Could you check a few things on this model? Use its own coordinates, in mm. Face numbers are marked on the shaded views. A direction names the side the tool comes from. Give positions to 0.01 mm unless a question says otherwise; leave off trailing zeros. Write each loop counter-clockwise with the first axis right and the second up, starting at its lowest first coordinate (ties: lowest second). Pieces come first, ordered by that corner, then holes. Notation, with made-up numbers: (40, -2) - (54, -2) arc R32 cw to (54, 34) - close; hole circle Ø5 at (-6, 86). An arc over 180 degrees is marked (long way). Answer in a Markdown table with one row per item.
from build123d import *

# Parameters (mm, degrees)
F2_R     = 4.7625
F2_R_2   = 1.5875
F5_DEPTH = 3.175
F6_DEPTH = 3.175
F4_W     = 7.239
F4_H     = 4.654424265
F7_DEPTH = 1.5875
F8_SIZE  = 0.79375


with BuildPart() as f5:
    # F2 (on offset) → F5 (new body, symmetric)
    with BuildSketch(Plane.XZ.offset(25.4)):
        Circle(F2_R)
        Circle(F2_R_2, mode=Mode.SUBTRACT)
    extrude(amount=F5_DEPTH, both=True)

    # F3 (on offset) → F6 (join, symmetric)
    with BuildSketch(Plane.XZ.offset(25.4)):
        with BuildLine():
            Line((3.175, 0), (3.175, 12.7))
            Line((3.175, 12.7), (-3.175, 12.7))
            Line((-3.175, 12.7), (-3.175, 0))
            Line((-3.175, 0), (-1.5875, 0))
            ThreePointArc((-1.5875, 0), (0, 1.5875), (1.5875, 0))
            Line((1.5875, 0), (3.175, 0))
        make_face()
    extrude(amount=F6_DEPTH, both=True)

    # F4 (on offset) → F7 (join, symmetric)
    with BuildSketch(Plane.XZ.offset(25.4)):
        with Locations((-5.5793230124, 8.6660822853)):
            Rectangle(F4_W, F4_H)
    extrude(amount=F7_DEPTH, both=True)

    # F8
    f8_edges = [f5.edges().sort_by_distance(p)[0] for p in [
        (0, -28.575, -4.7625),
        (0, -22.225, -4.7625),
    ]]
    chamfer(f8_edges, length=F8_SIZE)


solid = f5.part
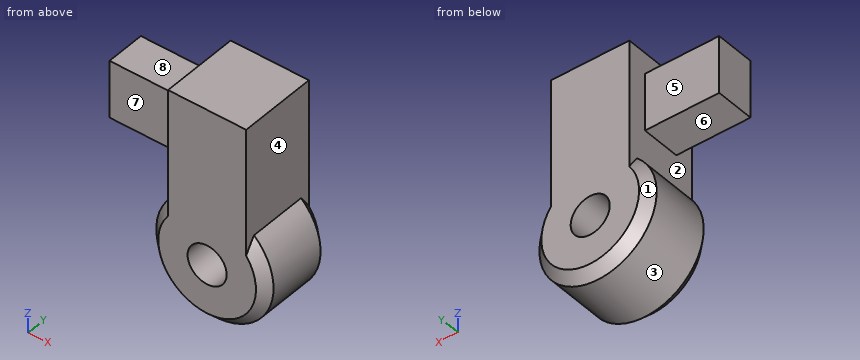
1) Will these pins go through, and if not, where does the flat tip stop? P1, Ø1.6, axis at x = -5, y = -25, coming from the -Z side; P2, Ø1.4, axis at x = -6, z = 8, coming from the +Y side; P3, Ø2.5, axis at x = -6, y = -25, coming from the +Z side; P4, Ø2.5, axis at x = 0, z = 0, coming from the +Y side.
Check values:
| item | result |
|---|---|
| P1 | stops at z = -2.25 |
| P2 | stops at y = -23.81 |
| P3 | stops at z = 10.99 |
| P4 | passes through |
2) On a 3-axis mill with a long thin cutter (end or side, diameter ignored), from which of +Z, -Z, +X, -X, +Y, -Y can I reach the whole of each face in a straight line? I mean the marked faces 5, 6, 7 and 8. Say none if no direction works.
Check values:
| item | result |
|---|---|
| face 5 | +Z, -X, +Y |
| face 6 | -X, +Y, -Y |
| face 7 | +Z, -X, -Y |
| face 8 | +Z, -X, +Y, -Y |
3) If I drill on line 1 (Z direction, x = 0, y = -25.75); line 2 (Z direction, x = -7.75, y = -24.75); line 3 (X direction, y = -25.75, z = 11.5) (3 decimals), over which ranges is the centre line in solid material (lowest first)?
Check values:
| item | result |
|---|---|
| line 1 | z = -4.76 to -1.59, 1.59 to 12.7 |
| line 2 | z = 6.34 to 10.99 |
| line 3 | x = -3.175 to 3.175 |
4) Imagine slicing it at B-B (y = -24). List the corners of the cut face in (x, z) for me (1 decimal).
Check values:
| item | result |
|---|---|
| outline | (-9.2, 6.3) - (-3.2, 6.3) - (-3.2, 3.5) arc R4.8 ccw (long way) to (3.2, 3.5) - (3.2, 12.7) - (-3.2, 12.7) - (-3.2, 11) - (-9.2, 11) - close; hole circle Ø3.2 at (0, 0) |
5) Imagine slicing it at C-C (x = 0). List the corners of the cut face in (y, z) for me (1 decimal), then the cut area to 3 significant figures.
Check values:
| item | result |
|---|---|
| outline | (-28.6, -4) - (-27.8, -4.8) - (-23, -4.8) - (-22.2, -4) - (-22.2, -1.6) - (-28.6, -1.6) - close; (-28.6, 1.6) - (-22.2, 1.6) - (-22.2, 12.7) - (-28.6, 12.7) - close |
| area | 90.1 mm2 |
6) Imagine slicing it at D-D (x = -7.25). List the corners of the cut face in (y, z) for me, then the cut area to 3 significant figures.
Check values:
| item | result |
|---|---|
| outline | (-26.99, 6.34) - (-23.81, 6.34) - (-23.81, 10.99) - (-26.99, 10.99) - close |
| area | 14.8 mm2 |
7) Imagine slicing it at A-A (z = 0). List the corners of the cut face in (x, y) for me (1 decimal).
Check values:
| item | result |
|---|---|
| outline | (-4.8, -27.8) - (-4, -28.6) - (-1.6, -28.6) - (-1.6, -22.2) - (-4, -22.2) - (-4.8, -23) - close; (1.6, -28.6) - (4, -28.6) - (4.8, -27.8) - (4.8, -23) - (4, -22.2) - (1.6, -22.2) - close |
8) We'd pull the mould along Z, two halves only. Please class the marked faces 1, 2, 3 and 4: +Z half, -Z half, draft (parallel to the pull), parting line (faces both ways), or undercut.
Check values:
| item | result |
|---|---|
| face 1 | parting line |
| face 2 | undercut |
| face 3 | undercut |
| face 4 | draft |
